```python
from build123d import *

# Parameters (mm, degrees)
EXTRUDE_1_DEPTH = 220
SKETCH_4_R      = 1
EXTRUDE_2_DEPTH = 15
SKETCH_5_R      = 2
EXTRUDE_3_DEPTH = 1
EXTRUDE_START   = 5
SKETCH_6_R      = 1
EXTRUDE_4_DEPTH = 5
EXTRUDE_START_2 = 1
SKETCH_7_R      = 2
EXTRUDE_5_DEPTH = 1


with BuildPart() as part:
    # 草图1 → 凸台-拉伸1 (new body)
    with BuildSketch(Plane(origin=(0, 0, 0), x_dir=(0, 0, -1), z_dir=(1, 0, 0))):
        Polygon((12.071067812, -5), (12.071067812, 5), (5, 12.071067812), (-5, 12.071067812), (-12.071067812, 5), (-12.071067812, -5), (-5, -12.071067812), (5, -12.071067812), align=None)
    extrude(amount=EXTRUDE_1_DEPTH)

    # 草图4 → 凸台-拉伸2 (add)
    with BuildSketch(Plane(origin=(220, 0, 0), x_dir=(0, 0, -1), z_dir=(1, 0, 0))):
        Circle(SKETCH_4_R)
    extrude(amount=EXTRUDE_2_DEPTH)

    # 草图5 → 凸台-拉伸3 (add)
    with BuildSketch(Plane(origin=(220, 0, 0), x_dir=(0, 0, -1), z_dir=(1, 0, 0))):
        Circle(SKETCH_5_R)
    extrude(amount=EXTRUDE_3_DEPTH)

    # 草图6 → 凸台-拉伸4 (add)
    with BuildSketch(Plane.ZY.offset(EXTRUDE_START)):
        with Locations(Location((0, 0, 0), (0, 0, 180))):
            Circle(SKETCH_6_R)
    extrude(amount=-EXTRUDE_4_DEPTH)

    # 草图7 → 凸台-拉伸5 (add)
    with BuildSketch(Plane.ZY.offset(EXTRUDE_START_2)):
        with Locations(Location((0, 0, 0), (0, 0, 180))):
            Circle(SKETCH_7_R)
    extrude(amount=-EXTRUDE_5_DEPTH)


solid = part.part
```
The model under review builds one solid part; all positions refer to its coordinate system, in mm. A direction names the side the tool comes from. Round coordinates to 2 decimals unless told otherwise and drop trailing zeros. Write each loop counter-clockwise with the first axis right and the second up, starting at its lowest first coordinate (ties: lowest second). Pieces come first, ordered by that corner, then holes. Notation, with made-up numbers: M 77,49.5 L 87,49.5 A17 ccw 87,67.5 Z; hole C -38,12 d9. An arc over 180 degrees is marked long. Use CSV: the item, a comma, the result in double quotes. Start each with the question number.
(1) Tool access review of faces 1 (the face through (-0.507, 1.952, 0.434)), 2 (the face through (221, -1, -1)), 3 (the face through (108, 12.071, 0)): name each direction out of +Z, -Z, +X, -X, +Y, -Y from which nothing blocks a thin tool from reaching the whole face with its end or side.
(2) For line 1 along X through (y, z) = (-3.25, -1.5); line 2 along Y through (x, z) = (218, 7.5); line 3 along Y through (x, z) = (183.5, -6.5), list the stretches that pass through material, from the lowest coordinate up.
(3) We need section B-B, the plane z = -9. State the section outline as (x, y) points.
(4) We need section A-A, the plane x = 190. State the section outline as (y, z) points.
(5) Clearance check with flat-ended pins moving along their axes: P1, Ø5, axis at y = 4, z = 5, coming from the +X side; P2, Ø5, axis at x = 183.5, y = 8, coming from the +Z side; P3, Ø12, axis at y = 9.5, z = 7.5, coming from the -X side. State where each tip first meets the part, or that it passes through.
(6) We need section C-C, the plane y = 7.5. State the section outline as (x, z) points, then the cut area to 3 significant figures.
Findings:
1,face 1,"-X"
1,face 2,"+X"
1,face 3,"+Z, -Z, +X, -X, +Y"
2,line 1,"0 to 220"
2,line 2,"-9.57 to 9.57"
2,line 3,"-10.57 to 10.57"
3,outline,"M 0,-8.07 L 220,-8.07 L 220,8.07 L 0,8.07 Z"
4,outline,"M -12.07,-5 L -5,-12.07 L 5,-12.07 L 12.07,-5 L 12.07,5 L 5,12.07 L -5,12.07 L -12.07,5 Z"
5,P1,"x = 220"
5,P2,"z = 11.57"
5,P3,"x = 0"
6,outline,"M 0,-9.57 L 220,-9.57 L 220,9.57 L 0,9.57 Z"
6,area,"4,210 mm^2"
